Verification items for the finished model (mm, model axes). Face numbers are marked on the shaded views. A direction names the side the tool comes from. Coordinates: 2 decimals unless noted, no trailing zeros. Order: outer loops, then holes, each group sorted by start corner. A loop starts at its lowest first (then second) coordinate and runs counter-clockwise, first axis right, second up. Notation, with made-up numbers: (38, 14) -> (72, 14) arc R29 ccw to (72, 44) -> close; hole circle Ø10 at (21.25, 31). An arc over 180 degrees is marked (long way). Write each question's results on one line, items separated by ' | '. Start each with the question number.
(1) Cross-section at B-B on y = 25.5. Enter the section's corners in (x, z).
(2) Go/stop test with flat-tipped pins: pin 1 (3.5 mm diameter, centred on x = 11, z = -21, fed in from -Y); pin 2 (1.8 mm diameter, centred on y = 55.5, z = -21, fed in from +X); pin 3 (14 mm diameter, centred on x = 97.5, z = -10, fed in from +Y); pin 4 (6.5 mm diameter, centred on y = 37.5, z = -14, fed in from -X). Record where each tip stops, or that it passes through.
(3) Cross-section at C-C on x = 151. Enter the section's corners in (y, z).
(4) Thickness scan on probe 1 along Z at (x, y) = (-0.4, 68.5); probe 2 along Z at (x, y) = (161, 1); probe 3 along X at (y, z) = (81.5, -7.5). Record the ranges inside material, lowest first. Write a range as [from, to].
(5) Cross-section at A-A on y = 37.5. Enter the section's corners in (x, z), and give its area (3 significant figures).
(6) Set-up check for the marked faces 1 and 2: record each of +Z, -Z, +X, -X, +Y, -Y from which the full face is reachable in a straight line by a thin tool's end or side.
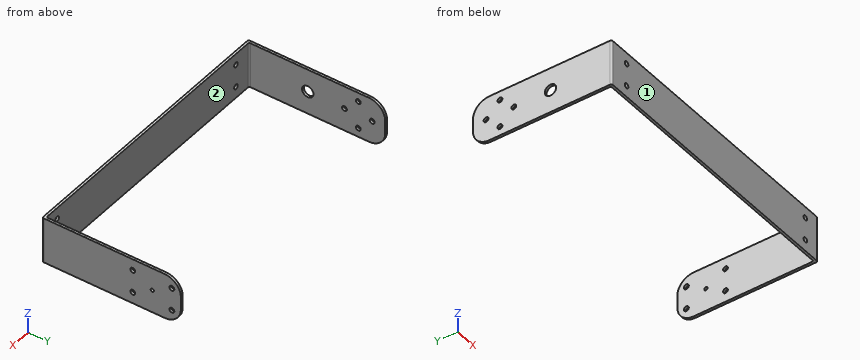
```python
from build123d import *

# Parameters (mm, degrees)
SKETCH1_W               = 170
SKETCH1_H               = 28
BOSS_EXTRUDE1_DEPTH     = 1.5
SKETCH2_W               = 28
SKETCH2_H               = 85
BOSS_EXTRUDE2_DEPTH     = 1.5
FILLET2_R               = 10
FILLET3_R               = 1
FILLET4_R               = 1
SKETCH5_R               = 1.5
CUT_EXTRUDE2_DEPTH      = 15
CUT_EXTRUDE2_DEPTH_BACK = 15
SKETCH7_R               = 3.5
CUT_EXTRUDE3_DEPTH      = 15
CUT_EXTRUDE3_DEPTH_BACK = 15
SKETCH8_R               = 1.5
CUT_EXTRUDE4_DEPTH      = 15
CUT_EXTRUDE4_DEPTH_BACK = 15
SKETCH11_W              = 28
SKETCH11_H              = 85
SKETCH11_R              = 1
BOSS_EXTRUDE5_DEPTH     = 1.5
FILLET5_R               = 1
FILLET6_R               = 1
FILLET7_R               = 10
FILLET8_R               = 10
SKETCH12_R              = 1.5
CUT_EXTRUDE5_DEPTH      = 10
CUT_EXTRUDE5_DEPTH_BACK = 10


with BuildPart() as part:
    # Sketch1 → Boss-Extrude1 (new body)
    with BuildSketch(Plane(origin=(0, 0, 0), x_dir=(1, 0, 0), z_dir=(0, 1, 0))):
        with Locations((85, 14)):
            Rectangle(SKETCH1_W, SKETCH1_H)
    extrude(amount=BOSS_EXTRUDE1_DEPTH)

    # Sketch2 → Boss-Extrude2 (add)
    with BuildSketch(Plane(origin=(0, 0, 0), x_dir=(0, 0, -1), z_dir=(1, 0, 0))):
        with Locations((14, 42.5)):
            Rectangle(SKETCH2_W, SKETCH2_H)
    extrude(amount=-BOSS_EXTRUDE2_DEPTH)

    # Fillet2
    fillet2_edges = [part.edges().sort_by_distance(p)[0] for p in [
        (-0.75, 85, -28),
        (-0.75, 85, 0),
    ]]
    fillet(fillet2_edges, radius=FILLET2_R)

    # Fillet3
    fillet3_edges = [part.edges().sort_by_distance(p)[0] for p in [
        (-1.5, 0, -14),
    ]]
    fillet(fillet3_edges, radius=FILLET3_R)

    # Fillet4
    fillet4_edges = [part.edges().sort_by_distance(p)[0] for p in [
        (0, 1.5, -14),
    ]]
    fillet(fillet4_edges, radius=FILLET4_R)

    # Sketch5 → Cut-Extrude2 (cut, two sides)
    with BuildSketch(Plane(origin=(0, 0, 0), x_dir=(0, 0, -1), z_dir=(1, 0, 0))) as cut_extrude2_sk:
        with Locations((14, 77)):
            Circle(SKETCH5_R)
        with Locations((14, 60)):
            Circle(SKETCH5_R)
        with Locations((22.5, 68.5)):
            Circle(SKETCH5_R)
        with Locations((5.5, 68.5)):
            Circle(SKETCH5_R)
    extrude(amount=CUT_EXTRUDE2_DEPTH, mode=Mode.SUBTRACT)
    extrude(cut_extrude2_sk.sketch, amount=-CUT_EXTRUDE2_DEPTH_BACK, mode=Mode.SUBTRACT)

    # Sketch7 → Cut-Extrude3 (cut, two sides)
    with BuildSketch(Plane(origin=(0, 0, 0), x_dir=(0, 0, -1), z_dir=(1, 0, 0))) as cut_extrude3_sk:
        with Locations((14, 37.5)):
            Circle(SKETCH7_R)
    extrude(amount=CUT_EXTRUDE3_DEPTH, mode=Mode.SUBTRACT)
    extrude(cut_extrude3_sk.sketch, amount=-CUT_EXTRUDE3_DEPTH_BACK, mode=Mode.SUBTRACT)

    # Sketch8 → Cut-Extrude4 (cut, two sides)
    with BuildSketch(Plane(origin=(0, 1.5, 0), x_dir=(1, 0, 0), z_dir=(0, 1, 0))) as cut_extrude4_sk:
        with Locations((161, 7)):
            Circle(SKETCH8_R)
        with Locations((11, 21)):
            Circle(SKETCH8_R)
        with Locations((11, 7)):
            Circle(SKETCH8_R)
        with Locations((161, 21)):
            Circle(SKETCH8_R)
    extrude(amount=CUT_EXTRUDE4_DEPTH, mode=Mode.SUBTRACT)
    extrude(cut_extrude4_sk.sketch, amount=-CUT_EXTRUDE4_DEPTH_BACK, mode=Mode.SUBTRACT)

    # Sketch11 → Boss-Extrude5 (add)
    with BuildSketch(Plane(origin=(170, 0, 0), x_dir=(0, 0, -1), z_dir=(1, 0, 0))):
        with Locations((14, 42.5)):
            Rectangle(SKETCH11_W, SKETCH11_H)
        with Locations((14, 67.5)):
            Circle(SKETCH11_R, mode=Mode.SUBTRACT)
    extrude(amount=BOSS_EXTRUDE5_DEPTH)

    # Fillet5
    fillet5_edges = [part.edges().sort_by_distance(p)[0] for p in [
        (170, 1.5, -14),
    ]]
    fillet(fillet5_edges, radius=FILLET5_R)

    # Fillet6
    fillet6_edges = [part.edges().sort_by_distance(p)[0] for p in [
        (171.5, 0, -14),
    ]]
    fillet(fillet6_edges, radius=FILLET6_R)

    # Fillet7
    fillet7_edges = [part.edges().sort_by_distance(p)[0] for p in [
        (170.75, 85, 0),
    ]]
    fillet(fillet7_edges, radius=FILLET7_R)

    # Fillet8
    fillet8_edges = [part.edges().sort_by_distance(p)[0] for p in [
        (170.75, 85, -28),
    ]]
    fillet(fillet8_edges, radius=FILLET8_R)

    # Sketch12 → Cut-Extrude5 (cut, two sides)
    with BuildSketch(Plane.ZY.offset(-170)) as cut_extrude5_sk:
        with Locations((-21, 79.5)):
            Circle(SKETCH12_R)
        with Locations((-7, 79.5)):
            Circle(SKETCH12_R)
        with Locations((-7, 55.5)):
            Circle(SKETCH12_R)
        with Locations((-21, 55.5)):
            Circle(SKETCH12_R)
    extrude(amount=CUT_EXTRUDE5_DEPTH, mode=Mode.SUBTRACT)
    extrude(cut_extrude5_sk.sketch, amount=-CUT_EXTRUDE5_DEPTH_BACK, mode=Mode.SUBTRACT)


solid = part.part
```
Results are:
1) outline: (-1.5, -28) -> (0, -28) -> (0, 0) -> (-1.5, 0) -> close; (170, -28) -> (171.5, -28) -> (171.5, 0) -> (170, 0) -> close
2) pin 1: stops at y = 0 | pin 2: stops at x = 0 | pin 3: stops at y = 1.5 | pin 4: stops at x = 170
3) outline: (0, -28) -> (1.5, -28) -> (1.5, 0) -> (0, 0) -> close
4) probe 1: z = [-28, -24], [-21, -7], [-4, 0] | probe 2: z = [-28, -22.5], [-19.5, -8.5], [-5.5, 0] | probe 3: x = [-1.5, 0], [170, 171.5]
5) outline: (-1.5, -28) -> (0, -28) -> (0, -17.5) -> (-1.5, -17.5) -> close; (-1.5, -10.5) -> (0, -10.5) -> (0, 0) -> (-1.5, 0) -> close; (170, -28) -> (171.5, -28) -> (171.5, 0) -> (170, 0) -> close | area: 73.5 mm2
6) face 1: +Z, -Z, +X, -X, -Y | face 2: +Z, -Z, +Y
